```python
from build123d import *

# Parameters (mm, degrees)
SKETCH1_W           = 25.4
SKETCH1_H           = 50.8
SKETCH1_W_2         = 19.05
SKETCH1_H_2         = 44.45
BOSS_EXTRUDE2_DEPTH = 1892.3
SKETCH2_R           = 3.175
CUT_EXTRUDE1_DEPTH  = 25.4
SKETCH3_R           = 3.175
CUT_EXTRUDE2_DEPTH  = 25.4
SKETCH4_R           = 6.35
CUT_EXTRUDE3_DEPTH  = 3.175
SKETCH5_R           = 6.35
CUT_EXTRUDE4_DEPTH  = 3.175


with BuildPart() as part:
    # Sketch1 → Boss-Extrude2 (new body)
    with BuildSketch(Plane(origin=(0, 0, 0), x_dir=(1, 0, 0), z_dir=(0, 1, 0))):
        Rectangle(SKETCH1_W, SKETCH1_H)
        Rectangle(SKETCH1_W_2, SKETCH1_H_2, mode=Mode.SUBTRACT)
    extrude(amount=BOSS_EXTRUDE2_DEPTH)

    # Sketch2 → Cut-Extrude1 (cut)
    with BuildSketch(Plane(origin=(12.7, 0, 0), x_dir=(0, 0, -1), z_dir=(1, 0, 0))):
        with Locations((12.7, 1844.658598875)):
            Circle(SKETCH2_R)
        with Locations((12.7, 1590.658598875)):
            Circle(SKETCH2_R)
        with Locations((12.7, 1336.658598875)):
            Circle(SKETCH2_R)
        with Locations((12.7, 1082.658598875)):
            Circle(SKETCH2_R)
        with Locations((12.7, 828.658598875)):
            Circle(SKETCH2_R)
        with Locations((12.7, 574.658598875)):
            Circle(SKETCH2_R)
        with Locations((12.7, 320.658598875)):
            Circle(SKETCH2_R)
    extrude(amount=-CUT_EXTRUDE1_DEPTH, mode=Mode.SUBTRACT)

    # Sketch3 → Cut-Extrude2 (cut)
    with BuildSketch(Plane(origin=(12.7, 0, 0), x_dir=(0, 0, -1), z_dir=(1, 0, 0))):
        with Locations((12.7, 117.458598875)):
            Circle(SKETCH3_R)
    extrude(amount=-CUT_EXTRUDE2_DEPTH, mode=Mode.SUBTRACT)

    # Sketch4 → Cut-Extrude3 (cut)
    with BuildSketch(Plane(origin=(12.7, 0, 0), x_dir=(0, 0, -1), z_dir=(1, 0, 0))):
        with Locations((12.7, 1844.658598875)):
            Circle(SKETCH4_R)
        with Locations((12.7, 1590.658598875)):
            Circle(SKETCH4_R)
        with Locations((12.7, 1336.658598875)):
            Circle(SKETCH4_R)
        with Locations((12.699999999, 1082.658598875)):
            Circle(SKETCH4_R)
        with Locations((12.699999999, 828.658598875)):
            Circle(SKETCH4_R)
        with Locations((12.699999999, 574.658598875)):
            Circle(SKETCH4_R)
        with Locations((12.699999999, 320.658598875)):
            Circle(SKETCH4_R)
    extrude(amount=-CUT_EXTRUDE3_DEPTH, mode=Mode.SUBTRACT)

    # Sketch5 → Cut-Extrude4 (cut)
    with BuildSketch(Plane(origin=(12.7, 0, 0), x_dir=(0, 0, -1), z_dir=(1, 0, 0))):
        with Locations((12.7, 117.458598875)):
            Circle(SKETCH5_R)
    extrude(amount=-CUT_EXTRUDE4_DEPTH, mode=Mode.SUBTRACT)


solid = part.part
```
Verification items for the finished model (mm, model axes). A direction names the side the tool comes from. Coordinates: 2 decimals unless noted, no trailing zeros. Write each loop counter-clockwise with the first axis right and the second up, starting at its lowest first coordinate (ties: lowest second). Pieces come first, ordered by that corner, then holes. Notation, with made-up numbers: M 21,45 L 71,45 A28 cw 71,84 Z; hole C 3.5,-34 d7. An arc over 180 degrees is marked long. Answer as a JSON object with one key per item and string values. Group by question number.
(1) Cross-section at A-A, the plane y = 1360. Record the cut outline in (x, z) (3 decimals).
(2) Material ranges on line 1 (X direction, y = 1145, z = -10) (3 decimals); line 2 (Z direction, x = 0, y = 573) (3 decimals), recorded low to high.
(3) Release check for a two-part mould opening along Z. For faces 1 (the face through (-9.525, 933, 0)), 2 (the face through (12.7, 933, 0)) record: +Z half, -Z half, draft (parallel to the pull), parting line (faces both ways), or undercut.
(4) Tool access check on faces 3 (the face through (9.525, 933, 0)), 4 (the face through (-12.7, 933, 0)). Record the directions out of +Z, -Z, +X, -X, +Y, -Y that give a thin tool (end or side, any length) a straight path to the whole face; none if there is none.
(5) Cross-section at B-B, the plane z = 7.5. Record the cut outline in (x, y) (3 decimals).
(6) Gauge pin test, flat ends, axial feed: pin 1 (5.5 mm diameter, centred on y = 320.66, z = -12.7, fed in from +X); pin 2 (10 mm diameter, centred on y = 117.46, z = -12.7, fed in from +X) (3 decimals). Record the tip position at first contact, or that the pin passes through.
Reply:
{
 "1": {"outline": "M -12.7,-25.4 L 12.7,-25.4 L 12.7,25.4 L -12.7,25.4 Z; hole M -9.525,-22.225 L 9.525,-22.225 L 9.525,22.225 L -9.525,22.225 Z"},
 "2": {"line 1": "-12.7 to -9.525, 9.525 to 12.7", "line 2": "-25.4 to -22.225, 22.225 to 25.4"},
 "3": {"face 1": "undercut", "face 2": "draft"},
 "4": {"face 3": "+Y, -Y", "face 4": "+Z, -Z, -X, +Y, -Y"},
 "5": {"outline": "M -12.7,0 L -9.525,0 L -9.525,1892.3 L -12.7,1892.3 Z; M 9.525,0 L 12.7,0 L 12.7,1892.3 L 9.525,1892.3 Z"},
 "6": {"pin 1": "through", "pin 2": "x = -9.525"}
}
